For this review, take the finished solid that the model builds, in its own axes (mm). Face numbers are marked on the shaded views. A direction names the side the tool comes from. Coordinates: 2 decimals unless noted, no trailing zeros. Order: outer loops, then holes, each group sorted by start corner. A loop starts at its lowest first (then second) coordinate and runs counter-clockwise, first axis right, second up.
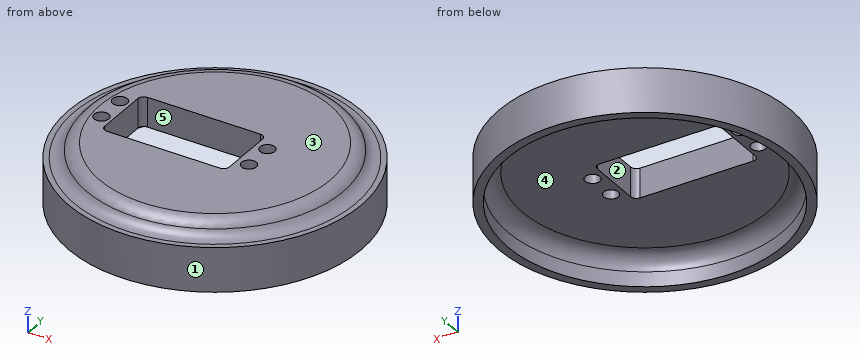
from build123d import *

# Parameters (mm, degrees)
SKETCH1_R           = 49.32
SKETCH1_R_2         = 46.32
EXTRUDE_THIN1_DEPTH = 10
SKETCH2_R           = 49.32
BOSS_EXTRUDE1_DEPTH = 5
SKETCH3_R           = 42.5
BOSS_EXTRUDE2_DEPTH = 5
FILLET1_R           = 5
FILLET2_R           = 5
SKETCH4_R           = 2.5
SKETCH4_W           = 42.1
SKETCH4_H           = 21.934824781
CUT_EXTRUDE1_DEPTH  = 73.559801543
FILLET3_R           = 2


with BuildPart() as part:
    # Sketch1 → Extrude-Thin1 (new body)
    with BuildSketch(Plane.XY):
        Circle(SKETCH1_R)
        Circle(SKETCH1_R_2, mode=Mode.SUBTRACT)
    extrude(amount=EXTRUDE_THIN1_DEPTH)

    # Sketch2 → Boss-Extrude1 (add)
    with BuildSketch(Plane.XY.offset(10)):
        Circle(SKETCH2_R)
    extrude(amount=BOSS_EXTRUDE1_DEPTH)

    # Sketch3 → Boss-Extrude2 (add)
    with BuildSketch(Plane.XY.offset(15)):
        Circle(SKETCH3_R)
    extrude(amount=BOSS_EXTRUDE2_DEPTH)

    # Fillet1
    fillet1_edges = [part.edges().sort_by_distance(p)[0] for p in [
        (-42.5, 0, 15),
        (-46.32, 0, 10),
    ]]
    fillet(fillet1_edges, radius=FILLET1_R - 0.0001)  # a hair under: the kernel refuses the full size

    # Fillet2
    fillet2_edges = [part.edges().sort_by_distance(p)[0] for p in [
        (-42.5, 0, 20),
    ]]
    fillet(fillet2_edges, radius=FILLET2_R)

    # Sketch4 → Cut-Extrude1 (cut, through all)
    with BuildSketch(Plane.XY.offset(20)):
        with Locations((-35.189613301, 5)):
            Circle(SKETCH4_R)
        with Locations((-35.189613301, -5)):
            Circle(SKETCH4_R)
        with Locations((14.589613301, 5)):
            Circle(SKETCH4_R)
        with Locations((14.589613301, -5)):
            Circle(SKETCH4_R)
        with Locations((-10.55, -0.067412391)):
            Rectangle(SKETCH4_W, SKETCH4_H)
    extrude(amount=-CUT_EXTRUDE1_DEPTH, mode=Mode.SUBTRACT)

    # Fillet3
    fillet3_edges = [part.edges().sort_by_distance(p)[0] for p in [
        (10.5, 10.9, 15),
        (10.5, -11.034824781, 15),
        (-31.6, -11.034824781, 15),
        (-31.6, 10.9, 15),
    ]]
    fillet(fillet3_edges, radius=FILLET3_R)


solid = part.part
1. The part is to be moulded in two halves that separate along Y. For the marked faces 1, 2 and 3, say which applies: +Y half, -Y half, draft (parallel to the pull), parting line (faces both ways), or undercut.
Answer below:
face 1: parting line
face 2: undercut
face 3: draft
2. Machinability: for the marked faces 4 and 5, which of the approach directions +Z, -Z, +X, -X, +Y, -Y give a long, thin tool a straight path to every point of the face, cutting with its end or side? Answer none if there is none.
Answer below:
face 4: -Z
face 5: +Z, -Z
3. Clearance check with flat-ended pins moving along their axes: pin 1 Ø8 at (y, z) = (25.5, 17) entering from +X; pin 2 Ø3 at (x, z) = (-2.5, 16) entering from -Y; pin 3 Ø8 at (x, z) = (12.5, 11) entering from +Y; pin 4 Ø8 at (x, y) = (-35.19, 5) entering from +Z. State where each tip first meets the part, or that it passes through.
Answer below:
pin 1: stops at x = 44.12
pin 2: stops at y = -49.3
pin 3: stops at y = 48.58
pin 4: stops at z = 20
4. To check wall thickness, follow L1, parallel to X at y = -3, z = 11; L2, parallel to Z at x = 18, y = -27.5; L3, parallel to Y at x = -12, z = 13.75. State the ranges of each line that lie inside material, in increasing order.
Answer below:
L1: x = -49.23 to -36.69, -33.69 to -31.6, 10.5 to 13.09, 16.09 to 49.23
L2: z = 10 to 20
L3: y = -47.84 to -11.03, 10.9 to 47.84
5. Take a section at A-A, the plane z = 3.5. Give the boundary of the cut face in (x, y).
Answer below:
outline: circle Ø98.64 at (0, 0); hole circle Ø92.64 at (0, 0)
6. Take a section at B-B, the plane y = -5. Give the number of separate pieces and of enclosed holes in the cut face, plus the area to 3 significant figures.
Answer below:
separate pieces: 4
enclosed holes: 0
area: 470 mm2
